Here's how the part is built. I have some questions about the finished solid (model axes, mm). A direction names the side the tool comes from. Round coordinates to 2 decimals unless told otherwise and drop trailing zeros. Order: outer loops, then holes, each group sorted by start corner. A loop starts at its lowest first (then second) coordinate and runs counter-clockwise, first axis right, second up. Notation, with made-up numbers: (-7, -39) - (42, -39) arc R21 ccw to (42, -26) - close; hole circle Ø1 at (89.25, 24). An arc over 180 degrees is marked (long way). One line per item, written item: value.
from build123d import *

# Parameters (mm, degrees)
SKETCH1_R           = 3.429
SKETCH1_R_2         = 2.286
BOSS_EXTRUDE1_DEPTH = 3.556
BOSS_EXTRUDE2_DEPTH = 1.27
BOSS_EXTRUDE3_START = -1.016
SKETCH2_3_R         = 2.286
SKETCH2_3_R_2       = 1.27
BOSS_EXTRUDE3_DEPTH = 0.254
SKETCH3_R           = 0.508
CUT_EXTRUDE1_DEPTH  = 17.020635974
LPATTERN1_COUNT     = 6
LPATTERN1_PITCH     = 1.778


with BuildPart() as part:
    # Sketch1 → Boss-Extrude1 (new body)
    with BuildSketch(Plane(origin=(0, 0, 0), x_dir=(1, 0, 0), z_dir=(0, 1, 0))):
        with Locations(Location((0, 0, 0), (0, 0, 270))):
            Circle(SKETCH1_R)
        with Locations(Location((0, 0, 0), (0, 0, 270))):
            Circle(SKETCH1_R_2, mode=Mode.SUBTRACT)
    extrude(amount=BOSS_EXTRUDE1_DEPTH)

    # Sketch2 → Boss-Extrude2 (add)
    with BuildSketch(Plane(origin=(0, 3.556, 0), x_dir=(1, 0, 0), z_dir=(0, 1, 0))):
        with BuildLine():
            ThreePointArc((-2.54, 2.303571358), (-1.389081498, 3.135042837), (0, 3.429))
            Line((0, 3.429), (0, 15.24))
            ThreePointArc((0, 15.24), (-0.835660201, 14.92028345), (-1.244511661, 14.124427226))
            Line((-1.244511661, 14.124427226), (-2.54, 2.303571358))
        make_face()
        with BuildLine():
            Line((0, 15.24), (0, 3.429))
            ThreePointArc((0, 3.429), (1.389081498, 3.135042837), (2.54, 2.303571358))
            Line((2.54, 2.303571358), (1.244511661, 14.124427226))
            ThreePointArc((1.244511661, 14.124427226), (0.835660201, 14.92028345), (0, 15.24))
        make_face()
    extrude(amount=-BOSS_EXTRUDE2_DEPTH)

    # Sketch2_3 → Boss-Extrude3 (add)
    with BuildSketch(Plane(origin=(0, 3.556, 0), x_dir=(1, 0, 0), z_dir=(0, 1, 0)).offset(BOSS_EXTRUDE3_START)):
        with Locations(Location((0, 0, 0), (0, 0, 270))):
            Circle(SKETCH2_3_R)
        with Locations(Location((0, 0, 0), (0, 0, 270))):
            Circle(SKETCH2_3_R_2, mode=Mode.SUBTRACT)
    extrude(amount=-BOSS_EXTRUDE3_DEPTH)

    # Sketch3 → Cut-Extrude1 (cut, through all)
    with BuildSketch(Plane(origin=(0, 3.556, 0), x_dir=(1, 0, 0), z_dir=(0, 1, 0))):
        with Locations(Location((0, 5.08, 0), (0, 0, 270))):
            Circle(SKETCH3_R)
    cut_extrude1 = extrude(amount=-CUT_EXTRUDE1_DEPTH, mode=Mode.SUBTRACT)

    # LPattern1: Cut-Extrude1 ×6
    with Locations(*[(0, 0, -i * LPATTERN1_PITCH) for i in range(1, LPATTERN1_COUNT)]):
        add(cut_extrude1, mode=Mode.SUBTRACT)


solid = part.part
Q1. We'd pull the mould along Z, two halves only. Please class faces 1 (the cylindrical face through (-0.31, 2.93, -9.04)), 2 (the flat face through (-1.883, 2.93, -8.297)), 3 (the flat face through (1, 2.286, -9)): released by +Z, released by -Z, zero draft, split by the parting line, or undercut.
Results list:
face 1: undercut
face 2: released by -Z
face 3: zero draft
Q2. If I drill on line 1 along Y through (x, z) = (-0.25, -14.5); line 2 along X through (y, z) = (2.9, 0.75); line 3 along X through (y, z) = (3.3, -12.5), over which ranges is the centre line in solid material (lowest first)?
Results list:
line 1: 2.29 to 3.56
line 2: -3.35 to -2.16, 2.16 to 3.35
line 3: -1.42 to -0.4, 0.4 to 1.42
Q3. Will these pins go through, and if not, where does the flat tip stop? pin 1 (1.3 mm diameter, centred on x = 0, z = -12.192, fed in from -Y); pin 2 (2 mm diameter, centred on y = 1.5, z = -6.5, fed in from +X); pin 3 (1.4 mm diameter, centred on x = 1, z = 0.5, fed in from +Y).
Results list:
pin 1: y = 2.29
pin 2: x = 2.15
pin 3: y = 2.54
Q4. Which directions (+Z, -Z, +X, -X, +Y, -Y) give clear straight access to the entire face, cutting with the end or side of a thin tool? Please do faces 4 (the flat face through (1.9, 2.93, -8.13)), 5 (the flat face through (-1.5, 2.286, 0)), 6 (the flat face through (-1.5, 2.54, 0)).
Results list:
face 4: -Z, +X, +Y, -Y
face 5: -Y
face 6: +Y
Q5. If we section it at A-A, the plane z = 0: Please give me the cut outline in (x, y), then the cut area to 3 significant figures.
Results list:
outline: (-3.43, 0) - (-2.29, 0) - (-2.29, 2.29) - (-1.27, 2.29) - (-1.27, 2.54) - (-2.29, 2.54) - (-2.29, 3.56) - (-3.43, 3.56) - close; (1.27, 2.29) - (2.29, 2.29) - (2.29, 0) - (3.43, 0) - (3.43, 3.56) - (2.29, 3.56) - (2.29, 2.54) - (1.27, 2.54) - close
area: 8.65 mm²
Q6. If we section it at B-B, the plane y = 3.2: Please give me the cut outline in (x, z), then the cut area to 3 significant figures.
Results list:
outline: (-2.54, -2.3) - (-1.24, -14.12) arc R1.25 ccw to (1.24, -14.12) - (2.54, -2.3) arc R3.43 ccw (long way) to start; hole circle Ø4.57 at (0, 0); hole circle Ø1.02 at (0, -13.97); hole circle Ø1.02 at (0, -12.19); hole circle Ø1.02 at (0, -10.41); hole circle Ø1.02 at (0, -8.64); hole circle Ø1.02 at (0, -6.86); hole circle Ø1.02 at (0, -5.08)
area: 58.6 mm²
Q7. If we section it at D-D, the plane y = 0.45: Please give me the cut outline in (x, z).
Results list:
outline: circle Ø6.86 at (0, 0); hole circle Ø4.57 at (0, 0)
Q8. If we section it at C-C, the plane x = 1: Please give me the cut outline in (y, z), then the cut area to 3 significant figures.
Results list:
outline: (0, -3.28) - (2.29, -3.28) - (2.29, -14.74) - (3.56, -14.74) - (3.56, -2.06) - (2.54, -2.06) - (2.54, -0.78) - (2.29, -0.78) - (2.29, -2.06) - (0, -2.06) - close; (0, 2.06) - (2.29, 2.06) - (2.29, 0.78) - (2.54, 0.78) - (2.54, 2.06) - (3.56, 2.06) - (3.56, 3.28) - (0, 3.28) - close
area: 23.9 mm²
